CAD build for the part. Positions are in the model's coordinates, mm. A direction names the side the tool comes from. Give positions to 0.01 mm unless a question says otherwise; leave off trailing zeros. Loops run counter-clockwise (first coordinate to the right, second up) from the corner with the lowest first, then second, coordinate; pieces in that order, holes last. Notation, with made-up numbers: M 19.25,9 L 46.25,9 A31 cw 46.25,42 Z; hole C 51.25,-14 d3. An arc over 180 degrees is marked long. Answer as CSV lines item,"result".
from build123d import *

# Parameters (mm, degrees)
SKETCH1_W                      = 12
SKETCH1_H                      = 10
BOSS_EXTRUDE1_DEPTH            = 3.5
CUT_EXTRUDE1_DEPTH             = 3.5
M2_5_CLEARANCE_HOLE1_D         = 2.7
M2_5_CLEARANCE_HOLE1_DEPTH     = 8.45
M2_5_TAPPED_HOLE1_D            = 2.05
M2_5_TAPPED_HOLE1_DEPTH        = 1
F_1_5_1_5_DIAMETER_HOLE1_D     = 1.5
F_1_5_1_5_DIAMETER_HOLE1_DEPTH = 3.5
M2_5_TAPPED_HOLE2_D            = 2.05
M2_5_TAPPED_HOLE4_D            = 2.05
M2_5_TAPPED_HOLE4_DEPTH        = 5
M2_5_TAPPED_HOLE4_TIP          = 0.615882135
M2_TAPPED_HOLE1_D              = 1.6


with BuildPart() as part:
    # Sketch1 → Boss-Extrude1 (new body)
    with BuildSketch(Plane(origin=(0, 0, 0), x_dir=(1, 0, 0), z_dir=(0, 1, 0))):
        Rectangle(SKETCH1_W, SKETCH1_H)
    extrude(amount=BOSS_EXTRUDE1_DEPTH)

    # Sketch2 → Cut-Extrude1 (cut)
    with BuildSketch(Plane(origin=(0, 3.5, 0), x_dir=(1, 0, 0), z_dir=(0, 1, 0))):
        with BuildLine():
            Line((2.777817459, -3.45), (2.176776695, -2.848959236))
            ThreePointArc((2.176776695, -2.848959236), (2, -2.775735931), (1.823223305, -2.848959236))
            Line((1.823223305, -2.848959236), (1.222182541, -3.45))
            Line((1.222182541, -3.45), (-1.75, -3.45))
            ThreePointArc((-1.75, -3.45), (-1.926776695, -3.523223305), (-2, -3.7))
            Line((-2, -3.7), (-2, -3.75))
            ThreePointArc((-2, -3.75), (-1.926776695, -3.926776695), (-1.75, -4))
            Line((-1.75, -4), (6, -4))
            Line((6, -4), (6, -3.45))
            Line((6, -3.45), (2.777817459, -3.45))
        make_face()
    extrude(amount=-CUT_EXTRUDE1_DEPTH, mode=Mode.SUBTRACT)

    # M2.5 Clearance Hole1
    with Locations(Plane(origin=(0, 0, -5), x_dir=(-1, 0, 0), z_dir=(0, 0, -1))):
        with Locations((-4.5, 1.75)):
            Hole(M2_5_CLEARANCE_HOLE1_D / 2, depth=M2_5_CLEARANCE_HOLE1_DEPTH)

    # M2.5 Tapped Hole1
    with Locations(Plane.XY.offset(5)):
        with Locations((4.5, 1.75)):
            Hole(M2_5_TAPPED_HOLE1_D / 2, depth=M2_5_TAPPED_HOLE1_DEPTH)

    # Ø1.5 (1.5) Diameter Hole1
    with Locations(Plane(origin=(0, 3.5, 0), x_dir=(1, 0, 0), z_dir=(0, 1, 0))):
        with Locations((-0.5, 1)):
            Hole(F_1_5_1_5_DIAMETER_HOLE1_D / 2, depth=F_1_5_1_5_DIAMETER_HOLE1_DEPTH)

    # M2.5 Tapped Hole2 (through all)
    with Locations(Plane(origin=(0, 0, -5), x_dir=(-1, 0, 0), z_dir=(0, 0, -1))):
        with Locations((0.5, 1.75)):
            Hole(M2_5_TAPPED_HOLE2_D / 2)

    # M2.5 Tapped Hole4
    with Locations(Plane.ZY.offset(6)):
        with Locations((-2.5, 1.75), (2.5, 1.75)):
            Hole(M2_5_TAPPED_HOLE4_D / 2, depth=M2_5_TAPPED_HOLE4_DEPTH)
            with Locations((0, 0, -(M2_5_TAPPED_HOLE4_DEPTH + M2_5_TAPPED_HOLE4_TIP / 2))):  # 118° drill point
                Cone(0, M2_5_TAPPED_HOLE4_D / 2, M2_5_TAPPED_HOLE4_TIP, mode=Mode.SUBTRACT)

    # M2 Tapped Hole1 (through all)
    with Locations(Plane(origin=(0, 0, 0), x_dir=(-1, 0, 0), z_dir=(0, -1, 0))):
        with Locations((-2, 0)):
            Hole(M2_TAPPED_HOLE1_D / 2)


solid = part.part
1) Mould opens along Y. For faces 1 (the face through (-1.4, 0.9, -5)), 2 (the face through (-3.46, 1.36, -3.45)), 3 (the face through (0, 0, 0)) say: +Y half, -Y half, draft (parallel to the pull), parting line (faces both ways), or undercut.
Answer below:
face 1,"draft"
face 2,"undercut"
face 3,"-Y half"
2) Drill centre lines: line 1 (Z direction, x = 2, y = 0.7); line 2 (Z direction, x = -0.5, y = 0.35); line 3 (Z direction, x = 5.75, y = 0.9). Where is each one in solid material? Low to high. Write a range as from..to.
Answer below:
line 1,"z = -5..-0.8, 0.8..2.78, 4..5"
line 2,"z = -5..-1.75, -0.25..3.45, 4..5"
line 3,"z = -5..3.45, 4..5"
3) Band-saw the part on B-B on x = 4.5. Give the cut face in (y, z) (3 decimals), and give its area (3 significant figures).
Answer below:
outline,"M 0,-5 L 0.4,-5 L 0.4,3.45 L 0,3.45 Z; M 0,4 L 0.725,4 L 0.725,5 L 0,5 Z; M 2.775,4 L 3.5,4 L 3.5,5 L 2.775,5 Z; M 3.1,-5 L 3.5,-5 L 3.5,3.45 L 3.1,3.45 Z"
area,"8.21 mm^2"
4) Band-saw the part on A-A on z = -1. Give the cut face in (x, y) (3 decimals), and give its area (3 significant figures).
Answer below:
outline,"M -6,0 L -1.25,0 L -1.25,1.051 A1.025 cw -1.25,2.449 L -1.25,3.5 L -6,3.5 Z; M 0.25,0 L 6,0 L 6,3.5 L 0.25,3.5 L 0.25,2.449 A1.025 cw 0.25,1.051 Z; hole C 4.5,1.75 d2.7"
area,"30.5 mm^2"
5) Band-saw the part on C-C on x = -3.5. Give the cut face in (y, z) (3 decimals).
Answer below:
outline,"M 0,-5 L 3.5,-5 L 3.5,5 L 0,5 Z; hole C 1.75,-2.5 d2.05; hole C 1.75,2.5 d2.05"
6) Which spindle directions (+Z, -Z, +X, -X, +Y, -Y) get a long thin tool onto all of the face, cutting with end or side? Do faces 4 (the face through (5.12, 0.55, -0.72)), 5 (the face through (-3.46, 1.36, 1.55)), 6 (the face through (1, 2, 3.45)). Say none if no direction does.
Answer below:
face 4,"-Z"
face 5,"-X"
face 6,"+X, +Y, -Y"
7) Band-saw the part on D-D on y = 1.75. Give the number of separate pieces and of enclosed holes in the cut face, and give its area (3 significant figures).
Answer below:
separate pieces,"7"
enclosed holes,"1"
area,"50.5 mm^2"
